Can you work these out from the model? Positions are in its coordinate system, mm. Face numbers are marked on the shaded views. Round coordinates to 2 decimals unless told otherwise and drop trailing zeros. Loops run counter-clockwise (first coordinate to the right, second up) from the corner with the lowest first, then second, coordinate; pieces in that order, holes last.
```python
from build123d import *

# Parameters (mm, degrees)
F0_W      = 50
F0_H      = 50
F1_DEPTH  = 50
F0_H_2    = 425
F2_DEPTH  = 25
F3_DEPTH  = 350
F5_DEPTH  = 50
F6_DEPTH  = 500
F8_DEPTH  = 50
F10_DEPTH = 50


with BuildPart() as f1:
    # F0 (on Top) → F1 (new body)
    with BuildSketch(Plane.XY):
        with Locations((-375, 475)):
            Rectangle(F0_W, F0_H)
    extrude(amount=F1_DEPTH)


with BuildPart() as f1b:
    # F0 (on Top) → F1, piece 2 (new body)
    with BuildSketch(Plane.XY):
        with Locations((-375, 0)):
            Rectangle(F0_W, F0_H)
    extrude(amount=F1_DEPTH)


with BuildPart() as f1c:
    # F0 (on Top) → F1, piece 3 (new body)
    with BuildSketch(Plane.XY):
        with Locations((375, 475)):
            Rectangle(F0_W, F0_H)
    extrude(amount=F1_DEPTH)


with BuildPart() as f1d:
    # F0 (on Top) → F1, piece 4 (new body)
    with BuildSketch(Plane.XY):
        with Locations((375, 0)):
            Rectangle(F0_W, F0_H)
    extrude(amount=F1_DEPTH)


with BuildPart() as f1e:
    # F0 (on Top) → F1, piece 5 (new body)
    with BuildSketch(Plane.XY):
        with Locations((-375, -475)):
            Rectangle(F0_W, F0_H)
    extrude(amount=F1_DEPTH)


with BuildPart() as f1f:
    # F0 (on Top) → F1, piece 6 (new body)
    with BuildSketch(Plane.XY):
        with Locations((375, -475)):
            Rectangle(F0_W, F0_H)
    extrude(amount=F1_DEPTH)


with BuildPart() as f2:
    # F0 (on Top) → F2 (new body)
    with BuildSketch(Plane.XY):
        with Locations((375, -475)):
            Rectangle(F0_W, F0_H)
        Polygon((-350, -500), (350, -500), (350, -450), (350, -25), (350, 25), (350, 450), (350, 500), (-350, 500), (-350, 450), (-350, 25), (-350, -25), (-350, -450), align=None)
        with Locations((375, -237.5)):
            Rectangle(F0_W, F0_H_2)
        with Locations((-375, -475)):
            Rectangle(F0_W, F0_H)
        with Locations((375, 0)):
            Rectangle(F0_W, F0_H)
        with Locations((-375, -237.5)):
            Rectangle(F0_W, F0_H_2)
        with Locations((375, 237.5)):
            Rectangle(F0_W, F0_H_2)
        with Locations((-375, 0)):
            Rectangle(F0_W, F0_H)
        with Locations((375, 475)):
            Rectangle(F0_W, F0_H)
        with Locations((-375, 237.5)):
            Rectangle(F0_W, F0_H_2)
        with Locations((-375, 475)):
            Rectangle(F0_W, F0_H)
    extrude(amount=F2_DEPTH)


with BuildPart() as f3:
    # F3 (new): a face of the model
    f3_faces = [f1e.part.faces().sort_by_distance(p)[0] for p in [
        (-375, -475, 50),
    ]]
    extrude(f3_faces, amount=F3_DEPTH)


with BuildPart() as f3b:
    # F3#2 (new): a face of the model
    f3_2_faces = [f1b.part.faces().sort_by_distance(p)[0] for p in [
        (-375, 0, 50),
    ]]
    extrude(f3_2_faces, amount=F3_DEPTH)


with BuildPart() as f3c:
    # F3#3 (new): a face of the model
    f3_3_faces = [f1.part.faces().sort_by_distance(p)[0] for p in [
        (-375, 475, 50),
    ]]
    extrude(f3_3_faces, amount=F3_DEPTH)


with BuildPart() as f3d:
    # F3#4 (new): a face of the model
    f3_4_faces = [f1c.part.faces().sort_by_distance(p)[0] for p in [
        (375, 475, 50),
    ]]
    extrude(f3_4_faces, amount=F3_DEPTH)


with BuildPart() as f3e:
    # F3#5 (new): a face of the model
    f3_5_faces = [f1d.part.faces().sort_by_distance(p)[0] for p in [
        (375, 0, 50),
    ]]
    extrude(f3_5_faces, amount=F3_DEPTH)


with BuildPart() as f3f:
    # F3#6 (new): a face of the model
    f3_6_faces = [f1f.part.faces().sort_by_distance(p)[0] for p in [
        (375, -475, 50),
    ]]
    extrude(f3_6_faces, amount=F3_DEPTH)


with BuildPart() as f3_1:
    add(f3.part)

    # F4: union F3b, F3c, F3d, F3e, F3f, F2, F1d, F1e, F1b, F1, F1c, F1f
    add(f3b.part)
    add(f3c.part)
    add(f3d.part)
    add(f3e.part)
    add(f3f.part)
    add(f2.part)
    add(f1d.part)
    add(f1e.part)
    add(f1b.part)
    add(f1.part)
    add(f1c.part)
    add(f1f.part)

    # F5 (add): faces of the model
    f5_faces = [f3_1.faces().sort_by_distance(p)[0] for p in [
        (375, 475, 400),
        (375, 0, 400),
        (375, -475, 400),
        (-375, -475, 400),
        (-375, 0, 400),
        (-375, 475, 400),
    ]]
    extrude(f5_faces, amount=F5_DEPTH)

    # F6 (add): faces of the model
    f6_faces = [f3_1.faces().sort_by_distance(p)[0] for p in [
        (-375, 0, 450),
        (375, 0, 450),
    ]]
    extrude(f6_faces, amount=F6_DEPTH)

    # F7 (on face) → F8 (join)
    with BuildSketch(Plane.YZ.offset(400)):
        Polygon((25, 500), (25, 450), (450, 450), (500, 450), (500, 500), align=None)
        Polygon((-500, 500), (-500, 450), (-450, 450), (-25, 450), (-25, 500), align=None)
    extrude(amount=-F8_DEPTH)

    # F9 (on face) → F10 (join)
    with BuildSketch(Plane(origin=(-400, 0, 0), x_dir=(0, -1, 0), z_dir=(-1, 0, 0))):
        Polygon((-500, 500), (-500, 450), (-450, 450), (-25, 450), (-25, 500), align=None)
        Polygon((25, 500), (25, 450), (450, 450), (500, 450), (500, 500), align=None)
    extrude(amount=-F10_DEPTH)


solid = f3_1.part
```
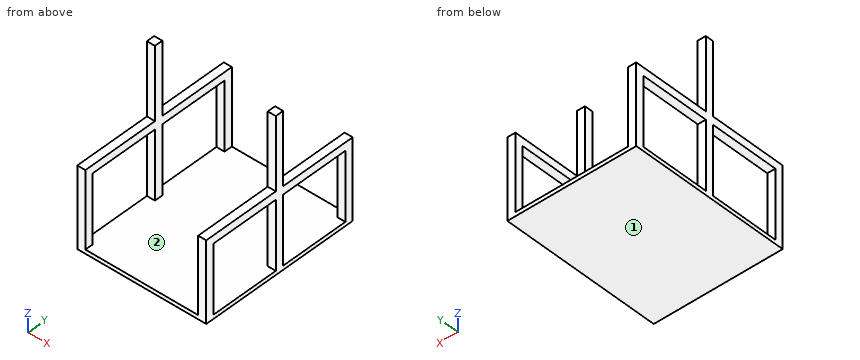
(1) Suppose I cut it at B-B (y = -434). Write out the boundary of the cut face in (x, z), then the cut area to 3 significant figures.
(2) We'd pull the mould along X, two halves only. Please class the marked faces 1 and 2: released by +X, released by -X, zero draft, split by the parting line, or undercut.
(3) For pin 1 (12 mm diameter, centred on x = 286, y = 336, fed in from +Z); pin 2 (15 mm diameter, centred on x = 373.5, y = -245.5, fed in from +Z); pin 3 (25 mm diameter, centred on x = -366.5, z = 764.5, fed in from -Y), each with a flat end and sliding along its axis, tell me the tip position at first contact or that it passes through.
(4) Suppose I cut it at A-A (z = 211). Write out the boundary of the cut face in (x, y), then the cut area to 3 significant figures.
(5) If I drill on line 1 (Z direction, x = -94, y = 363), over which ranges is the centre line in solid material (lowest first)?
(6) Suppose I cut it at C-C (z = 610.5). Write out the boundary of the cut face in (x, y), then the cut area to 3 significant figures.
(7) Suppose I cut it at D-D (x = 10.5). Write out the boundary of the cut face in (y, z).
Check result:
1. outline: (-400, 0) - (400, 0) - (400, 25) - (-400, 25) - close; (-400, 450) - (-350, 450) - (-350, 500) - (-400, 500) - close; (350, 450) - (400, 450) - (400, 500) - (350, 500) - close
1. area: 25,000 mm2
2. face 1: zero draft
2. face 2: undercut
3. pin 1: stops at z = 25
3. pin 2: stops at z = 500
3. pin 3: stops at y = -25
4. outline: (-400, -500) - (-350, -500) - (-350, -450) - (-400, -450) - close; (-400, -25) - (-350, -25) - (-350, 25) - (-400, 25) - close; (-400, 450) - (-350, 450) - (-350, 500) - (-400, 500) - close; (350, -500) - (400, -500) - (400, -450) - (350, -450) - close; (350, -25) - (400, -25) - (400, 25) - (350, 25) - close; (350, 450) - (400, 450) - (400, 500) - (350, 500) - close
4. area: 15,000 mm2
5. line 1: z = 0 to 25
6. outline: (-400, -25) - (-350, -25) - (-350, 25) - (-400, 25) - close; (350, -25) - (400, -25) - (400, 25) - (350, 25) - close
6. area: 5,000 mm2
7. outline: (-500, 0) - (500, 0) - (500, 25) - (-500, 25) - close
